For this review, take the finished solid that the model builds, in its own axes (mm). A direction names the side the tool comes from. Coordinates: 2 decimals unless noted, no trailing zeros. Order: outer loops, then holes, each group sorted by start corner. A loop starts at its lowest first (then second) coordinate and runs counter-clockwise, first axis right, second up.
from build123d import *

# Parameters (mm, degrees)
F1_DEPTH = 54
F2_R     = 4
F3_R     = 4
F6_DEPTH = 30
F7_D     = 5.5
F7_DEPTH = 25
F7_TIP   = 1.6523667023
F9_D     = 5.5
F9_DEPTH = 25
F9_TIP   = 1.6523667023


with BuildPart() as f1:
    # F0 (on Front) → F1 (new body)
    with BuildSketch(Plane.XZ):
        Polygon((0, 25), (0, 0), (40, 0), (40, 6), (6, 6), (6, 25), align=None)
    extrude(amount=F1_DEPTH)

    # F2
    f2_edges = [f1.edges().sort_by_distance(p)[0] for p in [
        (40, -27, 6),
    ]]
    fillet(f2_edges, radius=F2_R)

    # F3
    f3_edges = [f1.edges().sort_by_distance(p)[0] for p in [
        (6, -27, 6),
    ]]
    fillet(f3_edges, radius=F3_R)

    # F5 (on face) → F6 (cut)
    with BuildSketch(Plane(origin=(0, 0, 0), x_dir=(0, -1, 0), z_dir=(-1, 0, 0))):
        with BuildLine():
            Line((42.7775105486, 25), (11.508336102, 25))
            ThreePointArc((11.508336102, 25), (27.1429233253, 16.7962809503), (42.7775105486, 25))
        make_face()
        with BuildLine():
            ThreePointArc((42.7775105486, 25), (45.2820682506, 30.1419532821), (46.1429233253, 35.7962809503))
            ThreePointArc((46.1429233253, 35.7962809503), (21.4885956571, 53.9354258756), (11.508336102, 25))
            Line((11.508336102, 25), (42.7775105486, 25))
        make_face()
    extrude(amount=-F6_DEPTH, mode=Mode.SUBTRACT)

    # F7
    with Locations(Plane(origin=(0, 0, 0), x_dir=(0, 1, 0), z_dir=(-1, 0, 0))):
        with Locations((-8, -17), (-46, -17)):
            Hole(F7_D / 2, depth=F7_DEPTH)
            with Locations((0, 0, -(F7_DEPTH + F7_TIP / 2))):  # 118° drill point
                Cone(0, F7_D / 2, F7_TIP, mode=Mode.SUBTRACT)

    # F9
    with Locations(Plane(origin=(0, 0, 0), x_dir=(1, 0, 0), z_dir=(0, 0, -1))):
        with Locations((20, 46), (20, 8)):
            Hole(F9_D / 2, depth=F9_DEPTH)
            with Locations((0, 0, -(F9_DEPTH + F9_TIP / 2))):  # 118° drill point
                Cone(0, F9_D / 2, F9_TIP, mode=Mode.SUBTRACT)


solid = f1.part
1. Machinability: for faces 1 (the face through (3, -6, 25)), 2 (the face through (23, -27, 6)), which of the approach directions +Z, -Z, +X, -X, +Y, -Y give a long, thin tool a straight path to every point of the face, cutting with its end or side? Answer none if there is none.
Answer below:
face 1: +Z, +X, -X, +Y, -Y
face 2: +Z, +X, +Y, -Y
2. Take a section at B-B, the plane x = 20. Give the boundary of the cut face in (y, z).
Answer below:
outline: (-54, 0) - (-48.75, 0) - (-48.75, 6) - (-54, 6) - close; (-43.25, 0) - (-10.75, 0) - (-10.75, 6) - (-43.25, 6) - close; (-5.25, 0) - (0, 0) - (0, 6) - (-5.25, 6) - close
3. Take a section at A-A, the plane y = -46. Give the boundary of the cut face in (x, z), plus the area to 3 significant figures.
Answer below:
outline: (0, 0) - (17.25, 0) - (17.25, 6) - (10, 6) arc R4 cw to (6, 10) - (6, 14.25) - (0, 14.25) - close; (0, 19.75) - (6, 19.75) - (6, 25) - (0, 25) - close; (22.75, 0) - (40, 0) - (40, 2) arc R4 ccw to (36, 6) - (22.75, 6) - close
area: 288 mm2
4. To check wall thickness, follow L1, parallel to Y at x = 20, z = 1.75; L2, parallel to Z at x = 2.8, y = -46; L3, parallel to X at y = -27.5, z = 12.5. State the ranges of each line that lie inside material, in increasing order.
Answer below:
L1: y = -54 to -48.75, -43.25 to -10.75, -5.25 to 0
L2: z = 0 to 14.25, 19.75 to 25
L3: x = 0 to 6
5. Take a section at C-C, the plane x = 4. Give the boundary of the cut face in (y, z).
Answer below:
outline: (-54, 0) - (0, 0) - (0, 25) - (-11.51, 25) arc R19 cw to (-42.78, 25) - (-54, 25) - close; hole circle Ø5.5 at (-46, 17); hole circle Ø5.5 at (-8, 17)
6. Take a section at D-D, the plane y = -4.5. Give the boundary of the cut face in (x, z), plus the area to 3 significant figures.
Answer below:
outline: (0, 0) - (40, 0) - (40, 2) arc R4 ccw to (36, 6) - (10, 6) arc R4 cw to (6, 10) - (6, 25) - (0, 25) - close
area: 354 mm2
7. Clearance check with flat-ended pins moving along their axes: pin 1 Ø12 at (x, y) = (27, -15) entering from +Z; pin 2 Ø6 at (y, z) = (-37.5, 14) entering from -X; pin 3 Ø6.5 at (y, z) = (-46, 17) entering from +X. State where each tip first meets the part, or that it passes through.
Answer below:
pin 1: stops at z = 6
pin 2: stops at x = 0
pin 3: stops at x = 6
8. The part is to be moulded in two halves that separate along Y. For faces 3 (the face through (20.358, -48.727, 3.042)), 4 (the face through (7.203, -27.378, 7.141)), 5 (the face through (14, 0, 5)), say which applies: +Y half, -Y half, draft (parallel to the pull), parting line (faces both ways), or undercut.
Answer below:
face 3: undercut
face 4: draft
face 5: +Y half
